Source: three-view drawing plus pictorial views. Frame: mm from the lowest corner of the part. Coordinates: 2 decimals unless noted, no trailing zeros. Loops run counter-clockwise (first coordinate to the right, second up) from the corner with the lowest first, then second, coordinate; pieces in that order, holes last.
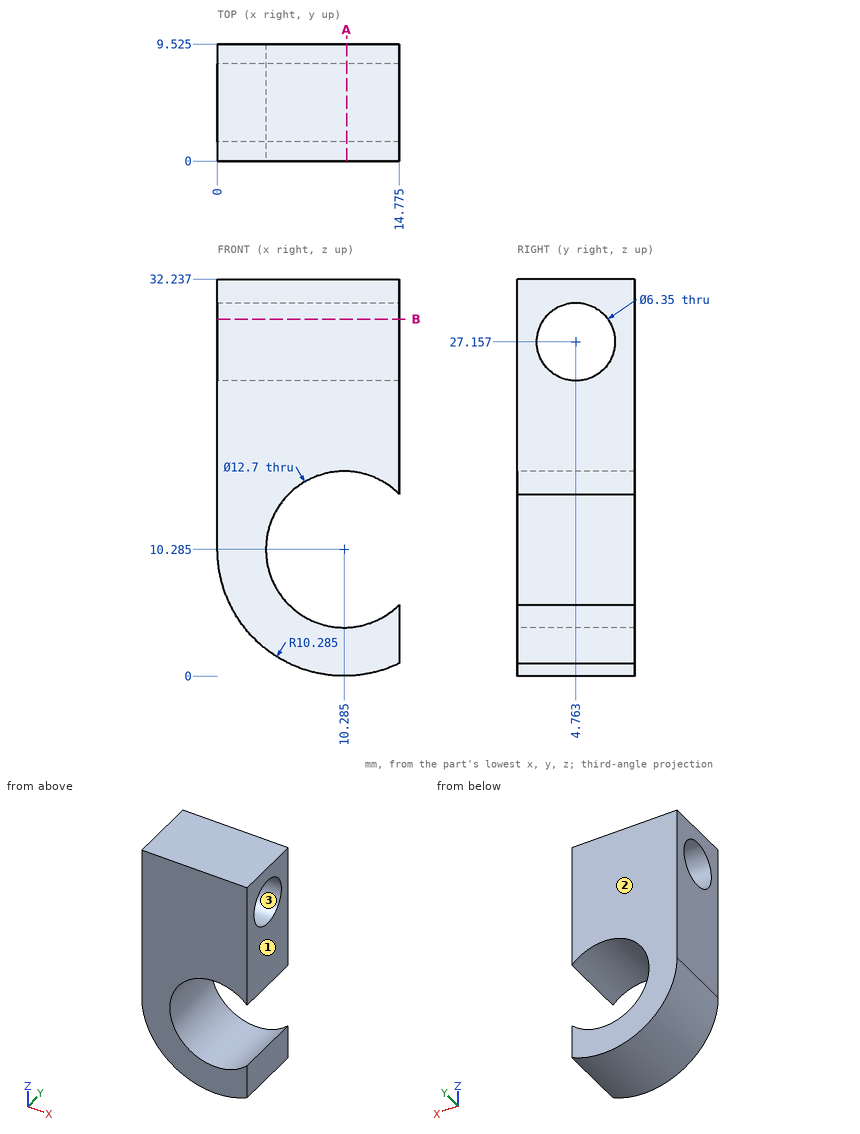
Q1. Material intervals for line 1 along Z through (x, y) = (9.5, 7) (1 decimal); line 2 along Z through (x, y) = (12.5, 5.5) (1 decimal); line 3 along Z through (x, y) = (3.5, 4) (1 decimal), sorted ascending.
Q2. Section query A-A on x = 10.5. Count the separate pieces of the cut face and the enclosed holes in it.
Q3. First-contact query: pin 1 Ø5 at (x, y) = (3.5, 3) entering from -Z (1 decimal). Flat tip, straight axial feed; report the tip coordinate or a pass-through.
Q4. Section query B-B on z = 29. Return the cut outline in (x, y) (1 decimal).
Q5. Draft query along Y for the marked faces 1, 2 and 3. Return one class per face: released by +Y, released by -Y, zero draft, split by the parting line, or undercut.
Resolved:
1. line 1: z = 0 to 4, 16.6 to 24.9, 29.4 to 32.2
1. line 2: z = 0.2 to 4.3, 16.2 to 24.1, 30.2 to 32.2
1. line 3: z = 2.6 to 24.1, 30.2 to 32.2
2. separate pieces: 2
2. enclosed holes: 1
3. pin 1: stops at z = 0.9
4. outline: (0, 0) - (14.8, 0) - (14.8, 2.2) - (0, 2.2) - close; (0, 7.3) - (14.8, 7.3) - (14.8, 9.5) - (0, 9.5) - close
5. face 1: zero draft
5. face 2: released by +Y
5. face 3: undercut
